from build123d import *

# Parameters (mm, degrees)
F1_DEPTH = 6.35
F3_DEPTH = 50.8
F5_D     = 13.49248
F6_R     = 19.05
F7_R     = 5.08
F8_R     = 5.08


# Not quite as in the source:
# - a feature names something its author has since deleted; it is built from what else it names


with BuildPart() as f1:
    # F0 (on Front) → F1 (new body)
    with BuildSketch(Plane.XZ):
        Polygon((37.9981123171, 180.8299914), (6.2481123171, 180.8299914), (6.2481123171, 60.2186896705), (-47.5612342455, 6.2650593709), (-20.5844190958, -20.6396139104), (0, 0), (6.2481123171, 0), (37.9981123171, 0), (37.9981123171, 33.02), align=None)
    extrude(amount=F1_DEPTH)

    # F2 (on face) → F3 (join)
    with BuildSketch(Plane(origin=(0, 0, 0), x_dir=(-1, 0, 0), z_dir=(0, 1, 0))):
        Polygon((52.0453464591, 1.7689235126), (47.5612342455, 6.2650593709), (20.5844190958, -20.6396139104), (25.0685313093, -25.1357497687), align=None)
    extrude(amount=-F3_DEPTH)

    # F5 (through all)
    with Locations(Plane.XZ.offset(6.35)):
        with Locations((22.2628123171, 118.2443914), (21.3484123171, 16.8009124652)):
            Hole(F5_D / 2)

    # F6
    f6_edges = [f1.edges().sort_by_distance(p)[0] for p in [
        (6.248112, -3.175, 60.21869),
        (37.998112, -3.175, 0),
        (0, -3.175, 0),
    ]]
    fillet(f6_edges, radius=F6_R)

    # F7
    f7_edges = [f1.edges().sort_by_distance(p)[0] for p in [
        (-38.556939, 0, -11.683413),
        (-34.072827, -6.35, -7.187277),
    ]]
    fillet(f7_edges, radius=F7_R)

    # F8
    f8_edges = [f1.edges().sort_by_distance(p)[0] for p in [
        (6.248112, -3.175, 180.829991),
        (37.998112, -3.175, 180.829991),
    ]]
    fillet(f8_edges, radius=F8_R)


solid = f1.part
Input: part model. Units: mm. Frame: model coordinates. A direction names the side the tool comes from. Round coordinates to 2 decimals unless told otherwise and drop trailing zeros. Loops run counter-clockwise (first coordinate to the right, second up) from the corner with the lowest first, then second, coordinate; pieces in that order, holes last. Notation, with made-up numbers: (-15, 14) -> (17, 14) arc R26 ccw to (17, 47) -> close; hole circle Ø4 at (39, 57.5). An arc over 180 degrees is marked (long way). Answer as a JSON object with one key per item and string values. Group by question number.
1) Section query C-C on y = -44.5. Output: boundary loops of the cut face in (x, z).
2) Section query B-B on z = 108. Output: boundary loops of the cut face in (x, y), plus the area to 3 significant figures.
3) Draft query along X for faces 5 (the cylindrical face through (18.636, -3.131, 123.933)), 6 (the flat face through (-36, -50.8, -9)), 7 (the cylindrical face through (32.27, -3.22, 5.43)). Return one class per face: +X half, -X half, draft (parallel to the pull), parting line (faces both ways), or undercut.
4) Section query A-A on y = -2.5. Output: boundary loops of the cut face in (x, z), plus the area to 3 significant figures.
5) Ray query, L1, parallel to Y at x = -24, z = -0.5; L2, parallel to Z at x = 25.5, y = -1.5. Return the intervals inside material, ascending.
6) Reachability of faces 1 (the flat face through (13, -3, 0)), 2 (the flat face through (-34.26, -30.84, -7)), 3 (the flat face through (6.248, -3, 123)), 4 (the flat face through (37.998, -3, 96)) from +Z, -Z, +X, -X, +Y, -Y: full face, straight path, thin tool, end or side. Return the list, or none.
7) Pin query (flat end, axial travel): pin 1 (1 mm diameter, centred on x = -24, y = -42.5, fed in from -Z); pin 2 (1.5 mm diameter, centred on x = 17.5, z = 78.5, fed in from -Y); pin 3 (3 mm diameter, centred on x = 13, y = -2.5, fed in from -Z); pin 4 (17.5 mm diameter, centred on x = 22.26, z = 118.24, fed in from +Y). Return the tip coordinate at first contact, or that it passes through.
Reply:
{
 "1": {"outline": "(-52.05, 1.77) -> (-25.07, -25.14) -> (-20.58, -20.64) -> (-47.56, 6.27) -> close"},
 "2": {"outline": "(6.25, -6.35) -> (38, -6.35) -> (38, 0) -> (6.25, 0) -> close", "area": "202 mm2"},
 "3": {"face 5": "undercut", "face 6": "draft", "face 7": "+X half"},
 "4": {"outline": "(-51.55, 2.27) -> (-24.57, -24.64) -> (-5.58, -5.6) arc R19.05 cw to (7.91, 0) -> (18.95, 0) arc R19.05 ccw to (38, 19.05) -> (38, 175.75) arc R5.08 ccw to (32.92, 180.83) -> (11.33, 180.83) arc R5.08 ccw to (6.25, 175.75) -> (6.25, 68.09) arc R19.05 cw to (0.69, 54.64) -> close; hole circle Ø13.49 at (21.35, 16.8); hole circle Ø13.49 at (22.26, 118.24)", "area": "7,790 mm2"},
 "5": {"L1": "y = -6.35 to 0", "L2": "z = 1.16 to 11.48, 22.12 to 112.33, 124.16 to 180.83"},
 "6": {"face 1": "-Z, +X, +Y, -Y", "face 2": "+Z, +X, -Y", "face 3": "+Z, -X, +Y, -Y", "face 4": "+Z, -Z, +X, +Y, -Y"},
 "7": {"pin 1": "stops at z = -24.57", "pin 2": "stops at y = -6.35", "pin 3": "stops at z = 0", "pin 4": "stops at y = 0"}
}
